Autodesk Fusion 360 part; units mm, degrees
sketch "Boceto1" plane through (0, 0, 0) normal (0, 0, 1) x (1, 0, 0)
  line L0 (0, 0) -> (0, 10) construction
  line L1 (55.2426, -86.6569) -> (49.1066, -86.6569)
  line L2 (0, -110.0711) -> (24, -110.0711)
  line L3 (24, -110.0711) -> (24, -103.0711)
  line L4 (24, -103.0711) -> (31.5563, -103.0711)
  line L5 (31.5563, -103.0711) -> (31.5563, -97.935)
  line L6 (31.5563, -97.935) -> (39.5563, -97.935)
  line L7 (39.5563, -97.935) -> (39.5563, -91.935)
  line L8 (39.5563, -91.935) -> (49.1066, -91.935)
  line L9 (49.1066, -91.935) -> (49.1066, -86.6569)
  line L10 (55.2426, -86.6569) -> (55.2426, 23.3431)
  line L11 (55.2426, 23.3431) -> (45.2426, 23.3431)
  line L12 (45.2426, 23.3431) -> (45.2426, 13.3431)
  line L13 (45.2426, 13.3431) -> (40.2426, 13.3431)
  line L14 (40.2426, 13.3431) -> (40.2426, 8.3431)
  line L15 (40.2426, 8.3431) -> (35.2426, 8.3431)
  line L16 (35.2426, 8.3431) -> (35.2426, 13.3431)
  line L17 (35.2426, 13.3431) -> (30.2426, 13.3431)
  line L18 (30.2426, 13.3431) -> (30.2426, 23.3431)
  line L19 (30.2426, 23.3431) -> (10.2426, 23.3431)
  line L20 (10.2426, 23.3431) -> (10.2426, 13.3431)
  line L21 (10.2426, 13.3431) -> (5.2426, 13.3431)
  line L22 (5.2426, 13.3431) -> (5.2426, 8.3431)
  line L23 (5.2426, 8.3431) -> (0, 8.3431)
  line L24 (0, -110.0711) -> (-24, -110.0711)
  line L25 (-24, -110.0711) -> (-24, -103.0711)
  line L26 (-24, -103.0711) -> (-31.5563, -103.0711)
  line L27 (-31.5563, -103.0711) -> (-31.5563, -97.935)
  line L28 (-31.5563, -97.935) -> (-39.5563, -97.935)
  line L29 (-39.5563, -97.935) -> (-39.5563, -91.935)
  line L30 (-39.5563, -91.935) -> (-49.1066, -91.935)
  line L31 (-49.1066, -91.935) -> (-49.1066, -86.6569)
  line L32 (-55.2426, -86.6569) -> (-49.1066, -86.6569)
  line L33 (-55.2426, -86.6569) -> (-55.2426, 23.3431)
  line L34 (-55.2426, 23.3431) -> (-45.2426, 23.3431)
  line L35 (-45.2426, 23.3431) -> (-45.2426, 13.3431)
  line L36 (-45.2426, 13.3431) -> (-40.2426, 13.3431)
  line L37 (-40.2426, 13.3431) -> (-40.2426, 8.3431)
  line L38 (-40.2426, 8.3431) -> (-35.2426, 8.3431)
  line L39 (-35.2426, 8.3431) -> (-35.2426, 13.3431)
  line L40 (-35.2426, 13.3431) -> (-30.2426, 13.3431)
  line L41 (-30.2426, 13.3431) -> (-30.2426, 23.3431)
  line L42 (-30.2426, 23.3431) -> (-10.2426, 23.3431)
  line L43 (-10.2426, 23.3431) -> (-10.2426, 13.3431)
  line L44 (-10.2426, 13.3431) -> (-5.2426, 13.3431)
  line L45 (-5.2426, 13.3431) -> (-5.2426, 8.3431)
  line L46 (-5.2426, 8.3431) -> (0, 8.3431)
  line L47 (-40.4532, -52.2423) -> (-36.5208, -52.2423) construction
  line L48 (-0.0272, -88.2631) -> (-23.5522, -88.2903)
  line L49 (-23.5522, -88.2903) -> (-30.6587, -81.1839)
  line L50 (-23.5522, -88.2903) -> (-13.5022, -88.2903) construction
  line L51 (-30.6587, -81.1839) -> (-35.7087, -81.1839)
  line L52 (-35.7087, -81.1839) -> (-40.6938, -76.1988)
  line L53 (-35.7087, -81.1839) -> (-28.6587, -81.1839) construction
  line L54 (-40.6938, -76.1988) -> (-40.6938, -52.1488)
  line L55 (-40.6938, -52.1488) -> (-37.83, -49.285)
  line L56 (-40.6938, -52.1488) -> (-36.6438, -52.1488) construction
  line L57 (-37.83, -49.285) -> (-37.83, -30.235)
  line L58 (-37.83, -30.235) -> (-29.3093, -21.7144)
  line L59 (-37.83, -30.235) -> (-25.78, -30.235) construction
  line L60 (-29.3093, -21.7144) -> (-29.3093, -14.6644)
  line L61 (-29.3093, -14.6644) -> (-27.1527, -12.5077)
  line L62 (-29.3093, -14.6644) -> (-26.2593, -14.6644) construction
  line L63 (-27.1527, -12.5077) -> (-27.1527, -6.4577)
  line L64 (-0.0272, -88.2631) -> (-0.0272, -6.4263) construction
  line L65 (-0.0272, -6.4263) -> (-27.1527, -6.4577)
  line L66 (-0.0272, -88.2631) -> (23.4977, -88.2903)
  line L67 (23.4977, -88.2903) -> (30.6042, -81.1839)
  line L68 (30.6042, -81.1839) -> (35.6542, -81.1839)
  line L69 (35.6542, -81.1839) -> (40.6393, -76.1988)
  line L70 (40.6393, -76.1988) -> (40.6393, -52.1488)
  line L71 (40.6393, -52.1488) -> (37.7755, -49.285)
  line L72 (37.7755, -49.285) -> (37.7755, -30.235)
  line L73 (37.7755, -30.235) -> (29.2548, -21.7144)
  line L74 (29.2548, -21.7144) -> (29.2548, -14.6644)
  line L75 (29.2548, -14.6644) -> (27.0982, -12.5077)
  line L76 (27.0982, -12.5077) -> (27.0982, -6.4577)
  line L77 (-0.0272, -6.4263) -> (27.0982, -6.4577)
  line L78 (0, -96.0218) -> (0, 0.9507) construction
  line L79 (0, -96.0218) -> (-25.935, -96.0218)
  line L80 (-25.935, -96.0218) -> (-34.5352, -87.4216)
  line L81 (-25.935, -96.0218) -> (-13.7725, -96.0218) construction
  line L82 (-34.5352, -87.4216) -> (-39.6602, -87.4216)
  line L83 (-39.6602, -87.4216) -> (-46.2203, -80.8614)
  line L84 (-39.6602, -87.4216) -> (-30.3827, -87.4216) construction
  line L85 (-46.2203, -80.8614) -> (-46.2203, -54.8264)
  line L86 (-46.2203, -54.8264) -> (-42.2102, -50.8163)
  line L87 (-46.2203, -54.8264) -> (-40.5491, -54.8264) construction
  line L88 (-42.2102, -50.8163) -> (-42.2102, -29.8813)
  line L89 (-42.2102, -29.8813) -> (-32.08, -19.7511)
  line L90 (-42.2102, -29.8813) -> (-27.8839, -29.8813) construction
  line L91 (-32.08, -19.7511) -> (-32.08, -9.5261)
  line L92 (-32.08, -9.5261) -> (-28.5798, -6.0259)
  line L93 (-32.08, -9.5261) -> (-27.13, -9.5261) construction
  line L94 (-28.5798, -6.0259) -> (-28.5798, 1.1391)
  line L95 (-28.5798, 1.1391) -> (0, 1.1391)
  line L96 (0, -96.0218) -> (25.935, -96.0218)
  line L97 (25.935, -96.0218) -> (34.5352, -87.4216)
  line L98 (34.5352, -87.4216) -> (39.6602, -87.4216)
  line L99 (39.6602, -87.4216) -> (46.2203, -80.8614)
  line L100 (46.2203, -80.8614) -> (46.2203, -54.8264)
  line L101 (46.2203, -54.8264) -> (42.2102, -50.8163)
  line L102 (42.2102, -50.8163) -> (42.2102, -29.8813)
  line L103 (42.2102, -29.8813) -> (32.08, -19.7511)
  line L104 (32.08, -19.7511) -> (32.08, -9.5261)
  line L105 (32.08, -9.5261) -> (28.5798, -6.0259)
  line L106 (28.5798, -6.0259) -> (28.5798, 1.1391)
  line L107 (28.5798, 1.1391) -> (0, 1.1391)
  point P0 (0, 4.7536)
  point P1 (0, 4.7536)
  point P2 (0, 4.7536)
  point P3 (0, -47.5355)
  point P4 (0, 2.3859)
  point P5 (0, 2.3859)
  point P6 (0, 2.3859)
  point P7 (0, -47.5355)
  point P8 (0, 0.9507)
  point P9 (0, -47.5355)
  point P10 (0, 0.9507)
  point P11 (0, -47.5355)
  point P12 (0, 0.9507)
  dimension "d46" = 24
  dimension "d48" = 7
  dimension "d49" = 8
  dimension "d50" = 6
  dimension "d52" = 110
  dimension "d53" = 10
  dimension "d54" = 10
  dimension "d55" = 5
  dimension "d56" = 5
  dimension "d57" = 5
  dimension "d58" = 5
  dimension "d59" = 5
  dimension "d60" = 10
  dimension "d61" = 20
  dimension "d62" = 10
  dimension "d63" = 5
  dimension "d64" = 5
  dimension "d144" = 135
  dimension "d145" = 10.05
  dimension "d146" = 5.05
  dimension "d147" = 135
  dimension "d148" = 7.05
  dimension "d149" = 24.05
  dimension "d150" = 4.05
  dimension "d151" = 45
  dimension "d152" = 19.05
  dimension "d153" = 45
  dimension "d154" = 12.05
  dimension "d155" = 7.05
  dimension "d156" = 3.05
  dimension "d157" = 45
  dimension "d158" = 6.05
  dimension "d168" = 135
  dimension "d169" = 12.1625
  dimension "d171" = 5.125
  dimension "d173" = 135
  dimension "d174" = 9.2775
  dimension "d176" = 26.035
  dimension "d178" = 5.6712
  dimension "d179" = 45
  dimension "d181" = 20.935
  dimension "d183" = 45
  dimension "d184" = 14.3262
  dimension "d186" = 10.225
  dimension "d188" = 4.95
  dimension "d189" = 45
  dimension "d191" = 7.165
ref_plane "PlanoDeObra1" through (55.2426, 23.3431, 35) normal (1, 0, 0) x (0, 1, 0)
sketch "Boceto2" plane through (55.2426, 0, 0) normal (1, 0, 0) x (0, 1, 0)
  line L0 (23.1427, -0.0591) -> (-6.8573, -0.0187)
  line L1 (-6.8573, -0.0187) -> (-6.8573, 32.9813)
  line L2 (-6.8573, 32.9813) -> (-36.8573, 32.9813)
  line L3 (-36.8573, 32.9813) -> (-36.8573, 4.9813)
  line L4 (-36.8573, 4.9813) -> (-6.8573, 4.9813)
  dimension "d198" = 30
  dimension "d200" = 30
  dimension "d201" = 28
extrude "Extruir16" add sketch "Boceto1" along normal blind 5 contours L48 L49 L51 L52 L54 L55 L57 L58 L60 L61 L63 L65 L66 L67 L68 L69 L70 L71 L72 L73 L74 L75 L76 L77
extrude "Extruir17" add sketch "Boceto1" along normal blind 32 contours L79 L80 L82 L83 L85 L86 L88 L89 L91 L92 L94 L95 L96 L97 L98 L99 L100 L101 L102 L103 L104 L105 L106 L107
extrude "Extruir18" add sketch "Boceto1" along normal blind 40 contours L1 L2 L3 L4 L5 L6 L7 L8 L9 L10 L11 L12 L13 L14 L15 L16 L17 L18 L19 L20 L21 L22 L23 L24 L25 L26 L27 L28 L29 L30 L31 L32 L33 L34 L35 L36 L37 L38 L39 L40 L41 L42 L43 L44 L45 L46
extrude "Extruir19" cut sketch "Boceto2" along normal mid plane 60
equation "d169 = 12.13748388 mm + 0.025 mm"
equation "d171 = 5.10 mm + 0.025 mm"
equation "d174 = 9.25248834 mm + 0.025 mm"
equation "d176 = 26.01 mm + 0.025 mm"
equation "d178 = 5.64624366 mm + 0.025 mm"
equation "d181 = 20.91 mm + 0.025 mm"
equation "d184 = 14.3012313 mm + 0.025 mm"
equation "d186 = 10.20 mm + 0.025 mm"
equation "d188 = 4.92499554 mm + 0.025 mm"
equation "d191 = 7.14 mm + 0.025 mm"
Design review of the part built by this model. Coordinates are the model's own, in mm. A direction names the side the tool comes from. Round coordinates to 2 decimals unless told otherwise and drop trailing zeros. Loops run counter-clockwise (first coordinate to the right, second up) from the corner with the lowest first, then second, coordinate; pieces in that order, holes last. Notation, with made-up numbers: (-33, -35) -> (4, -35) arc R15 ccw to (4, -16) -> close; hole circle Ø1 at (56, 36). An arc over 180 degrees is marked (long way). Use one line per item in the form item = value. Start each with the question number.
Q1. Machinability: for faces 1 (the face through (-43, 13.343, 20)), 2 (the face through (-38.166, -78.726, 18.311)), 3 (the face through (-33.629, -26.034, 18.311)), 4 (the face through (-31.556, -101, 20)), 5 (the face through (31.556, -101, 20)), which of the approach directions +Z, -Z, +X, -X, +Y, -Y give a long, thin tool a straight path to every point of the face, cutting with its end or side? Answer none if there is none.
Q2. For pin 1 Ø5 at (x, z) = (-41, 33) entering from +Y; pin 2 Ø3 at (x, z) = (-2.5, 27.5) entering from +Y; pin 3 Ø1 at (x, y) = (-16.5, -74) entering from -Z; pin 4 Ø1 at (y, z) = (-89, 26) entering from +X, all flat-tipped, find the tip position at first contact; note any pin that passes through.
Q3. We need section C-C on y = -42. Give the boundary of the cut face in (x, z).
Q4. We need section A-A on y = 15.5. Give the boundary of the cut face in (x, z), then the cut area to 3 significant figures.
Q5. Draft analysis for pull direction X (two halves, no side actions). For faces 6 (the face through (44.243, -52.849, 35.944)), 7 (the face through (-39.556, -95, 20)), 8 (the face through (-52, -86.657, 20)), state which applies: +X half, -X half, draft (parallel to the pull), parting line (faces both ways), or undercut.
Q6. We need section D-D on x = -2.5. Give the boundary of the cut face in (y, z), then the cut area to 3 significant figures.
Q7. Wall thickness on line 1 along X through (y, z) = (13, 16); line 2 along Y through (x, z) = (16, 7); line 3 along X through (y, z) = (-59, 27.5): over which ranges is each line inside the solid? List them lowest first. Write a range as [from, to].
Calculated:
q1.face_1 = +Z, -Z, +Y
q1.face_2 = +Z
q1.face_3 = +Z, +X
q1.face_4 = +Z, -Z, -X, -Y
q1.face_5 = +Z, -Z, +X, -Y
q2.pin_1 = 13.34
q2.pin_2 = 8.34
q2.pin_3 = 0
q2.pin_4 = 49.11
q3.outline = (-55.24, 0) -> (55.24, 0) -> (55.24, 40) -> (42.21, 40) -> (42.21, 32) -> (37.78, 32) -> (37.78, 5) -> (-37.83, 5) -> (-37.83, 32) -> (-42.21, 32) -> (-42.21, 40) -> (-55.24, 40) -> close
q4.outline = (-55.24, 0) -> (-45.24, 0) -> (-45.24, 40) -> (-55.24, 40) -> close; (-30.24, 0) -> (-10.24, 0) -> (-10.24, 40) -> (-30.24, 40) -> close; (10.24, 0) -> (30.24, 0) -> (30.24, 40) -> (10.24, 40) -> close; (45.24, 0) -> (55.24, 0) -> (55.24, 40) -> (45.24, 40) -> close
q4.area = 2,400 mm²
q5.face_6 = undercut
q5.face_7 = -X half
q5.face_8 = draft
q6.outline = (-110.07, 0) -> (8.34, 0) -> (8.34, 40) -> (1.14, 40) -> (1.14, 32) -> (-6.43, 32) -> (-6.43, 5) -> (-88.27, 5) -> (-88.27, 32) -> (-96.02, 32) -> (-96.02, 40) -> (-110.07, 40) -> close
q6.area = 1,750 mm²
q7.line_1 = [-55.24, -40.24], [-35.24, -5.24], [5.24, 35.24], [40.24, 55.24]
q7.line_2 = [-110.07, -88.28], [-6.44, 23.34]
q7.line_3 = [-55.24, -40.69], [40.64, 55.24]
